Study the drawing (mm; zero at the part's minimum x, y, z) and answer. Coordinates: 2 decimals unless noted, no trailing zeros. Loops run counter-clockwise (first coordinate to the right, second up) from the corner with the lowest first, then second, coordinate; pieces in that order, holes last. Notation, with made-up numbers: (20, 86.25) - (59, 86.25) arc R8 cw to (59, 101.25) - close; hole circle Ø5 at (51, 51). An arc over 180 degrees is marked (long way). Write each question's results on one line, items separated by ' | '. Start each with the question number.
(1) Consider line 1 (X direction, y = 2.55, z = 5); line 2 (X direction, y = 3, z = 57.4); line 3 (Z direction, x = 242, y = 3.3). Determine where each line is inside the solid, lowest interval first. Write a range as from..to.
(2) Find section B-B on z = 35. Determine the outline of the cut face in (x, y), then the cut area to 3 significant figures.
(3) Find section A-A on y = 3.55. State how many separate pieces and enclosed holes the cut face has, then the cut area to 3 significant figures.
(4) Given pin 1 Ø3 at (x, y) = (147, 3.5) entering from +Z; pin 2 Ø2.5 at (x, y) = (115, 3.5) entering from -Z; pin 3 Ø2.5 at (x, z) = (166.5, 5) entering from +Y; pin 4 Ø2.5 at (y, z) = (3, 14.5) entering from +X, each flat-ended and moving along its own axis, determine where each tip first touches the part or whether it passes through.
(5) Find section C-C on x = 41. Determine the outline of the cut face in (y, z).
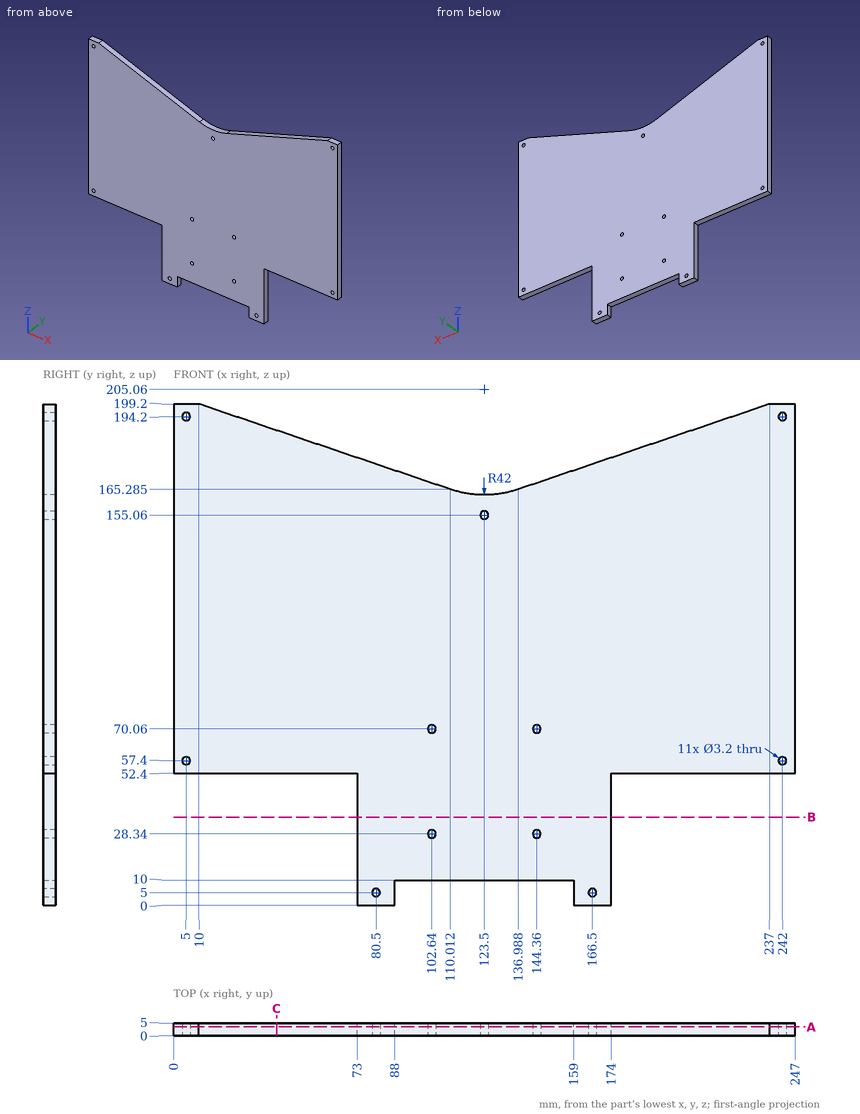
Values:
1) line 1: x = 73..78.9, 82.1..88, 159..164.9, 168.1..174 | line 2: x = 0..3.4, 6.6..240.4, 243.6..247 | line 3: z = 52.4..55.8, 59..192.6, 195.8..199.2
2) outline: (73, 0) - (174, 0) - (174, 5) - (73, 5) - close | area: 505 mm²
3) separate pieces: 1 | enclosed holes: 11 | area: 36,400 mm²
4) pin 1: stops at z = 169.19 | pin 2: stops at z = 10 | pin 3: passes through | pin 4: stops at x = 174
5) outline: (0, 52.4) - (5, 52.4) - (5, 188.69) - (0, 188.69) - close
